For this review, use the dimensioned drawing (mm, ordinates from the lowest corner) and the shaded views. Coordinates: 2 decimals unless noted, no trailing zeros. Write each loop counter-clockwise with the first axis right and the second up, starting at its lowest first coordinate (ties: lowest second). Pieces come first, ordered by that corner, then holes.
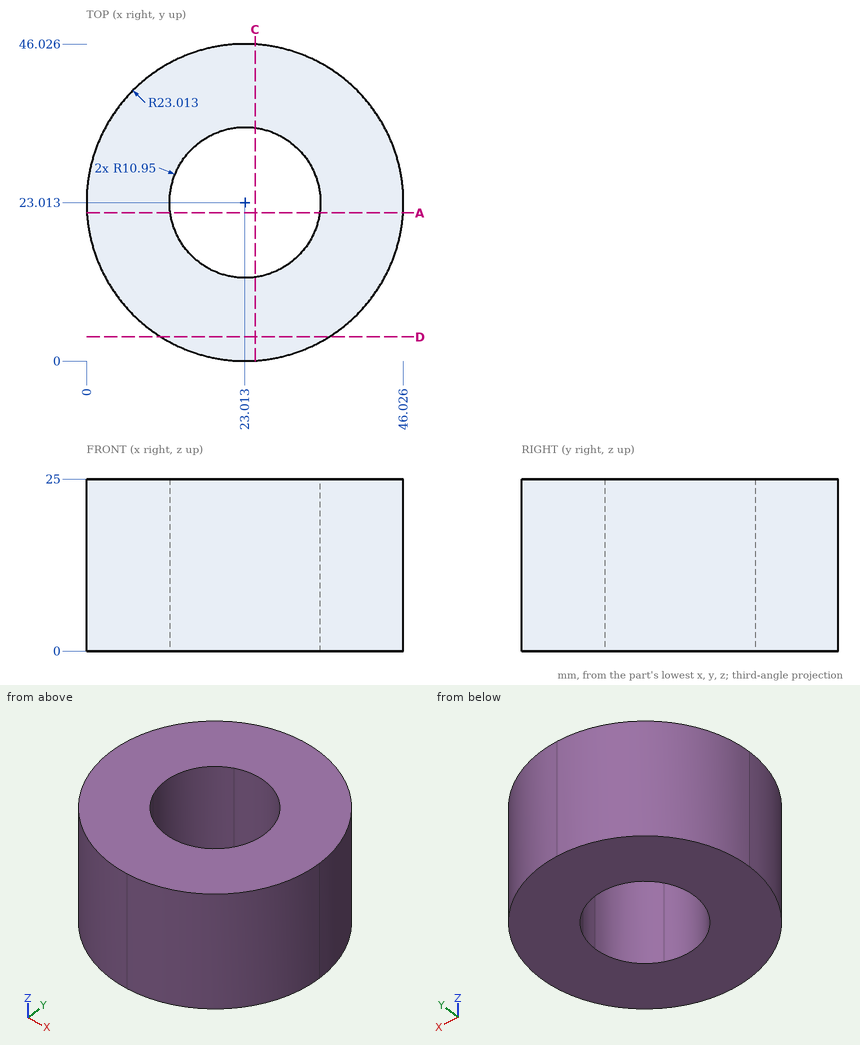
Item 1: Take a section at C-C, the plane x = 24.5. Write out the cut boundary in (y, z).
Solved:
outline: (0.05, 0) - (12.16, 0) - (12.16, 25) - (0.05, 25) - close; (33.86, 0) - (45.98, 0) - (45.98, 25) - (33.86, 25) - close
Item 2: To check wall thickness, follow line 1 along Y through (x, z) = (24, 14.5) (1 decimal); line 2 along Y through (x, z) = (32.5, 8.75) (1 decimal); line 3 along X through (y, z) = (30.5, 21.5) (1 decimal). State the ranges of each line that lie inside material, in increasing order.
Solved:
line 1: y = 0 to 12.1, 33.9 to 46
line 2: y = 2 to 17.5, 28.5 to 44
line 3: x = 1.3 to 15, 31 to 44.8
Item 3: For pin 1 (5 mm diameter, centred on y = 35, z = 8, fed in from +X); pin 2 (1.5 mm diameter, centred on y = 24.5, z = 21, fed in from +X); pin 3 (2 mm diameter, centred on y = 12, z = 15, fed in from +X), all flat-tipped, find the tip position at first contact; note any pin that passes through.
Solved:
pin 1: stops at x = 43.98
pin 2: stops at x = 46.01
pin 3: stops at x = 43.73
Item 4: Take a section at D-D, the plane y = 3.5. Write out the cut boundary in (x, z), plus the area to 3 significant figures.
Solved:
outline: (10.81, 0) - (35.21, 0) - (35.21, 25) - (10.81, 25) - close
area: 610 mm2
Item 5: Take a section at A-A, the plane y = 21.5. Write out the cut boundary in (x, z).
Solved:
outline: (0.05, 0) - (12.17, 0) - (12.17, 25) - (0.05, 25) - close; (33.86, 0) - (45.98, 0) - (45.98, 25) - (33.86, 25) - close
